The drawing under review shows one solid part. Ordinate dimensions are in mm from its lowest x, y, z. Round coordinates to 2 decimals unless told otherwise and drop trailing zeros. Order: outer loops, then holes, each group sorted by start corner. A loop starts at its lowest first (then second) coordinate and runs counter-clockwise, first axis right, second up. Notation, with made-up numbers: (59.25, 89.25) - (69.25, 89.25) arc R19 ccw to (69.25, 124.25) - close; hole circle Ø4 at (70, 60.25). An arc over 180 degrees is marked (long way). One line per question, with ' | ' between items.
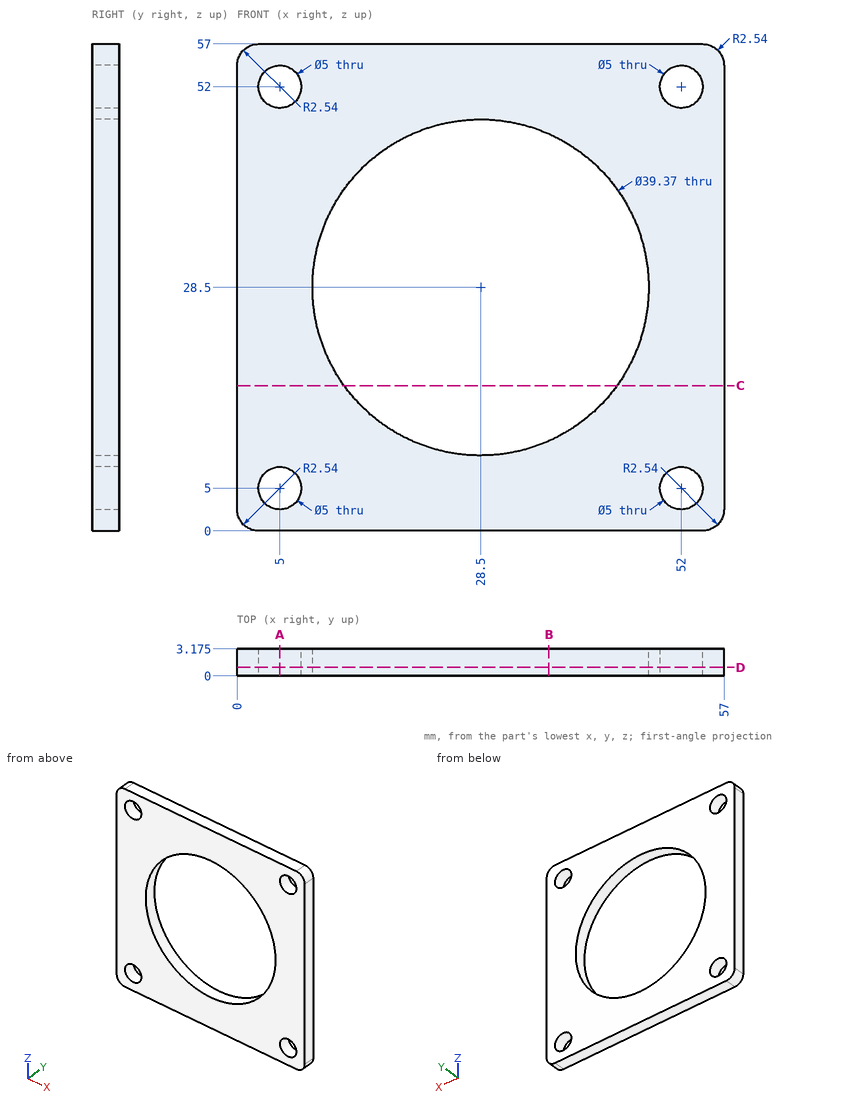
(1) We need section B-B on x = 36.5. State the section outline as (y, z) points (3 decimals).
Output values:
outline: (0, 0) - (3.175, 0) - (3.175, 10.514) - (0, 10.514) - close; (0, 46.486) - (3.175, 46.486) - (3.175, 57) - (0, 57) - close
(2) We need section A-A on x = 5. State the section outline as (y, z) points (3 decimals).
Output values:
outline: (0, 0) - (3.175, 0) - (3.175, 2.5) - (0, 2.5) - close; (0, 7.5) - (3.175, 7.5) - (3.175, 49.5) - (0, 49.5) - close; (0, 54.5) - (3.175, 54.5) - (3.175, 57) - (0, 57) - close
(3) We need section D-D on y = 1. State the section outline as (x, z) points (3 decimals).
Output values:
outline: (0, 2.54) arc R2.54 ccw to (2.54, 0) - (54.46, 0) arc R2.54 ccw to (57, 2.54) - (57, 54.46) arc R2.54 ccw to (54.46, 57) - (2.54, 57) arc R2.54 ccw to (0, 54.46) - close; hole circle Ø5 at (5, 5); hole circle Ø5 at (5, 52); hole circle Ø39.37 at (28.5, 28.5); hole circle Ø5 at (52, 5); hole circle Ø5 at (52, 52)
(4) For probe 1 along X at (y, z) = (1.55, 5); probe 2 along Z at (x, y) = (53.5, 1.7); probe 3 along Z at (x, y) = (5.5, 1.6), list the stretches that pass through material, from the lowest coordinate up. Write a range as [from, to].
Output values:
probe 1: [0, 2.5], [7.5, 49.5], [54.5, 57] | probe 2: [0, 3], [7, 50], [54, 57] | probe 3: [0, 2.55], [7.45, 49.55], [54.45, 57]
(5) Insertion check: pin 1 (1.5 mm diameter, centred on x = 31.5, z = 11, fed in from +Y). The pin has a flat end and moves straight along its axis. Give the tip position at first contact, or say it passes through.
Output values:
pin 1: through
(6) We need section C-C on z = 17. State the section outline as (x, y) points (1 decimal).
Output values:
outline: (0, 0) - (12.5, 0) - (12.5, 3.2) - (0, 3.2) - close; (44.5, 0) - (57, 0) - (57, 3.2) - (44.5, 3.2) - close
